from build123d import *

# Parameters (mm, degrees)
CUT_EXTRUDE_1_DEPTH = 5


with BuildPart() as part:
    # 草图4 → 旋转3 (revolve)
    with BuildSketch(Plane.XY, mode=Mode.PRIVATE) as revolve_3_sk:
        with BuildLine():
            Line((0, 0), (0, 32.8))
            Line((0, 32.8), (4.65, 32.8))
            ThreePointArc((4.65, 32.8), (5.357106781, 32.507106781), (5.65, 31.8))
            Line((5.65, 31.8), (5.65, 25))
            Line((5.65, 25), (3.738374166, 25))
            Line((3.738374166, 25), (3.3, 24.690748957))
            Line((3.3, 24.690748957), (4, 24.196933978))
            Line((4, 24.196933978), (3.3, 23.703118999))
            Line((3.3, 23.703118999), (4, 23.20930402))
            Line((4, 23.20930402), (3.3, 22.715489041))
            Line((3.3, 22.715489041), (4, 22.221674062))
            Line((4, 22.221674062), (3.3, 21.727859083))
            Line((3.3, 21.727859083), (4, 21.234044103))
            Line((4, 21.234044103), (3.3, 20.740229124))
            Line((3.3, 20.740229124), (4, 20.246414145))
            Line((4, 20.246414145), (3.3, 19.752599166))
            Line((3.3, 19.752599166), (4, 19.258784187))
            Line((4, 19.258784187), (3.3, 18.764969208))
            Line((3.3, 18.764969208), (4, 18.271154229))
            Line((4, 18.271154229), (3.3, 17.777339249))
            Line((3.3, 17.777339249), (4, 17.28352427))
            Line((4, 17.28352427), (3.3, 16.789709291))
            Line((3.3, 16.789709291), (4, 16.295894312))
            Line((4, 16.295894312), (3.3, 15.802079333))
            Line((3.3, 15.802079333), (4, 15.308264354))
            Line((4, 15.308264354), (3.3, 14.814449374))
            Line((3.3, 14.814449374), (4, 14.320634395))
            Line((4, 14.320634395), (3.3, 13.826819416))
            Line((3.3, 13.826819416), (4, 13.333004437))
            Line((4, 13.333004437), (3.3, 12.839189458))
            Line((3.3, 12.839189458), (4, 12.345374479))
            Line((4, 12.345374479), (3.3, 11.8515595))
            Line((3.3, 11.8515595), (4, 11.35774452))
            Line((4, 11.35774452), (3.3, 10.863929541))
            Line((3.3, 10.863929541), (4, 10.370114562))
            Line((4, 10.370114562), (3.3, 9.876299583))
            Line((3.3, 9.876299583), (4, 9.382484604))
            Line((4, 9.382484604), (3.3, 8.888669625))
            Line((3.3, 8.888669625), (4, 8.394854646))
            Line((4, 8.394854646), (3.3, 7.901039666))
            Line((3.3, 7.901039666), (4, 7.407224687))
            Line((4, 7.407224687), (3.3, 6.913409708))
            Line((3.3, 6.913409708), (4, 6.419594729))
            Line((4, 6.419594729), (3.3, 5.92577975))
            Line((3.3, 5.92577975), (4, 5.431964771))
            Line((4, 5.431964771), (3.3, 4.938149791))
            Line((3.3, 4.938149791), (4, 4.444334812))
            Line((4, 4.444334812), (3.3, 3.950519833))
            Line((3.3, 3.950519833), (4, 3.456704854))
            Line((4, 3.456704854), (3.3, 2.962889875))
            Line((3.3, 2.962889875), (4, 2.469074896))
            Line((4, 2.469074896), (3.3, 1.975259917))
            Line((3.3, 1.975259917), (4, 1.481444937))
            Line((4, 1.481444937), (3.3, 0.987629958))
            Line((3.3, 0.987629958), (4, 0.493814979))
            Line((4, 0.493814979), (3.3, 0))
            Line((3.3, 0), (0, 0))
        make_face()
    revolve(revolve_3_sk.sketch.rotate(Axis((0, 24.690748957, 0), (0, 1, 0)), 90), axis=Axis((0, 24.690748957, 0), (0, 1, 0)))

    # 草图6 → 切除-拉伸1 (cut)
    with BuildSketch(Plane(origin=(0, 32.8, 0), x_dir=(1, 0, 0), z_dir=(0, 1, 0))):
        Polygon((4.041451884, 0), (2.020725942, 3.5), (-2.020725942, 3.5), (-4.041451884, 0), (-2.020725942, -3.5), (2.020725942, -3.5), align=None)
    extrude(amount=-CUT_EXTRUDE_1_DEPTH, mode=Mode.SUBTRACT)


solid = part.part
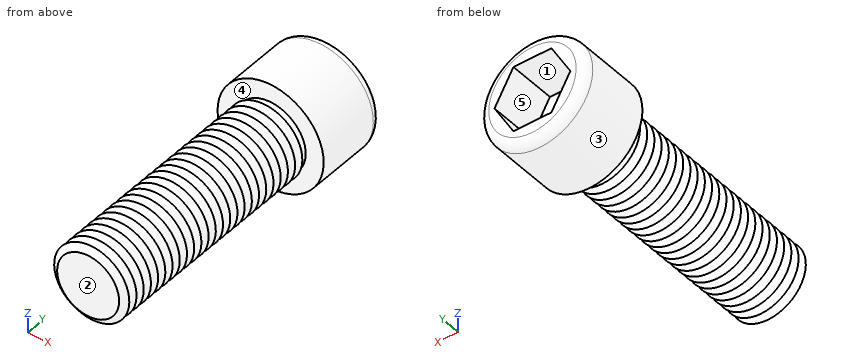
For this review, take the finished solid that the model builds, in its own axes (mm). Face numbers are marked on the shaded views. A direction names the side the tool comes from. Round coordinates to 2 decimals unless told otherwise and drop trailing zeros. Use a Markdown table: item, result. Add a question column.
Item 1: Mouldability with a two-part tool opening along X and no side actions: class the marked faces 1, 2 and 3 as released by +X, released by -X, zero draft, split by the parting line, or undercut.
Item 2: To check wall thickness, follow line 1 along Z through (x, y) = (-0.25, 30); line 2 along Y through (x, z) = (-4.25, 1.25); line 3 along Y through (x, z) = (-2.5, -2). State the ranges of each line that lie inside material, in increasing order.
Item 3: Insertion check: pin 1 (2 mm diameter, centred on x = 1.5, z = -1.5, fed in from +Y); pin 2 (1.2 mm diameter, centred on x = 1, y = 29.5, fed in from -Z); pin 3 (3 mm diameter, centred on x = 0, y = 14, fed in from +Z). Each pin has a flat end and moves straight along its axis. Give the tip position at first contact, or say it passes through.
Item 4: Tool access review of the marked faces 4 and 5: name each direction out of +Z, -Z, +X, -X, +Y, -Y from which nothing blocks a thin tool from reaching the whole face with its end or side.
Geometry results:
| question | item | result |
|---|---|---|
| 1 | face 1 | undercut |
| 1 | face 2 | zero draft |
| 1 | face 3 | split by the parting line |
| 2 | line 1 | z = -5.64 to -3.5, 3.5 to 5.64 |
| 2 | line 2 | y = 25 to 32.8 |
| 2 | line 3 | y = 0 to 27.8 |
| 3 | pin 1 | stops at y = 27.8 |
| 3 | pin 2 | stops at z = -5.64 |
| 3 | pin 3 | stops at z = 4 |
| 4 | face 4 | none |
| 4 | face 5 | +Y |
